Build history of the part. All positions in model axes, mm. Coordinates: 2 decimals unless noted, no trailing zeros. Loops run counter-clockwise (first coordinate to the right, second up) from the corner with the lowest first, then second, coordinate; pieces in that order, holes last.
(1) Wall check: L1, parallel to Y at x = -1, z = 13; L2, parallel to X at y = -12, z = 0.75; L3, parallel to X at y = 9.5, z = 4.5. Give the ranges that are in metal, low to high.
(2) Slice it at C-C (z = 7). Give the cut face in (x, y).
(3) Two-plate mould, pull along Y, no slides. Class faces 1 (the face through (-59.94, 2.64, 7.4)), 2 (the face through (12, -12, 0)), 3 (the face through (-35.326, 37.94, 7.605)): pulls with the +Y half, pulls with the -Y half, needs draft (parallel to the pull), parting line crosses it, or undercut.
(4) Slice it at D-D (x = 38.5). Give the cut face in (y, z), and give its area (3 significant figures).
(5) Flat gauge pins, fed straight in: P1, Ø1, axis at y = -37.5, z = 12, coming from the +X side; P2, Ø5, axis at y = -46, z = 10.5, coming from the -X side; P3, Ø3, axis at y = 42, z = 6.5, coming from the -X side; P4, Ø12, axis at x = -27.96, y = 31.18, coming from the -Z side. Where does each tip first touch, or does it go through?
(6) Slice it at A-A (y = 0). Give the cut face in (x, z), and give its area (3 significant figures).
from build123d import *

# Parameters (mm, degrees)
SKETCH1_R           = 60
BOSS_EXTRUDE1_DEPTH = 15
SKETCH3_R           = 15
CUT_EXTRUDE1_DEPTH  = 15
SKETCH4_R           = 10
CUT_EXTRUDE2_DEPTH  = 15


with BuildPart() as part:
    # Sketch1 → Boss-Extrude1 (new body)
    with BuildSketch(Plane.XY):
        Circle(SKETCH1_R)
    extrude(amount=BOSS_EXTRUDE1_DEPTH)

    # Sketch3 → Cut-Extrude1 (cut)
    with BuildSketch(Plane.XY.offset(15)):
        Circle(SKETCH3_R)
    extrude(amount=-CUT_EXTRUDE1_DEPTH, mode=Mode.SUBTRACT)

    # Sketch4 → Cut-Extrude2 (cut)
    with BuildSketch(Plane.XY.offset(15)):
        with Locations((-27.955634388, 31.181284509)):
            Circle(SKETCH4_R)
    extrude(amount=-CUT_EXTRUDE2_DEPTH, mode=Mode.SUBTRACT)


solid = part.part
Response values:
1. L1: y = -59.99 to -14.97, 14.97 to 59.99
1. L2: x = -58.79 to -9, 9 to 58.79
1. L3: x = -59.24 to -11.61, 11.61 to 59.24
2. outline: circle Ø120 at (0, 0); hole circle Ø20 at (-27.96, 31.18); hole circle Ø30 at (0, 0)
3. face 1: parting line crosses it
3. face 2: needs draft
3. face 3: undercut
4. outline: (-46.02, 0) - (46.02, 0) - (46.02, 15) - (-46.02, 15) - close
4. area: 1,380 mm2
5. P1: stops at x = 47.23
5. P2: stops at x = -41.32
5. P3: stops at x = -44.27
5. P4: passes through
6. outline: (-60, 0) - (-15, 0) - (-15, 15) - (-60, 15) - close; (15, 0) - (60, 0) - (60, 15) - (15, 15) - close
6. area: 1,350 mm2
